Autodesk Inventor part; units mm, degrees
ref_plane "bolt_to_nut_XY" through (8, 0, 0) normal (1, 0, 0) x (0, 0, -1)
ref_plane "bolt_to_nut_YZ" through (8, 0, 0) normal (0, 0, -1) x (0, 1, 0)
ref_plane "bolt_to_nut_ZX" through (8, 0, 0) normal (0, 1, 0) x (1, 0, 0)
sketch "Sketch_1" plane through (0, 0, 0) normal (0, 0, 1) x (1, 0, 0)
  line L0 (8, 0) -> (-5, 0)
  line L1 (-5, 0) -> (-5, 3.75)
  line L2 (-5, 3.75) -> (-4.5, 4.25)
  line L3 (-4.5, 4.25) -> (0, 4.25)
  line L4 (0, 4.25) -> (0, 2.5)
  line L5 (0, 2.5) -> (7.5095, 2.5)
  line L6 (7.5095, 2.5) -> (8, 2.0095)
  line L7 (8, 2.0095) -> (8, 0)
  line L8 (8, 0) -> (-5, 0)
revolve "Revolution1" add sketch "Sketch_1" angle 360 about axis through (8, 0, 0) along (1, 0, 0)
thread "Thread1"
sketch "Sketch2" plane through (-5, 0, 0) normal (-1, 0, 0) x (0, 0, 1)
  point P0 (0, 0)
hole "Hole1" at (-5, 0, 0) direction (1, 0, 0) diameter 4 depth 2.5 tip angle 150
sketch "Sketch_3" plane through (-5, 0, 0) normal (1, 0, 0) x (0, 0, -1)
  line L0 (-2, -1.1547) -> (0, -2.3094)
  line L1 (0, -2.3094) -> (2, -1.1547)
  line L2 (2, -1.1547) -> (2, 1.1547)
  line L3 (2, 1.1547) -> (0, 2.3094)
  line L4 (0, 2.3094) -> (-2, 1.1547)
  line L5 (-2, 1.1547) -> (-2, -1.1547)
extrude "Extrusion1" cut sketch "Sketch_3" along normal blind 2.5
ref_plane "bolt_to_nut_XY" through (8, 0, 0) normal (1, 0, 0) x (0, 0, -1)
ref_plane "bolt_to_nut_YZ" through (8, 0, 0) normal (0, 0, -1) x (0, 1, 0)
ref_plane "bolt_to_nut_ZX" through (8, 0, 0) normal (0, 1, 0) x (1, 0, 0)
ref_plane "screw1_XY" through (0, 0, 0) normal (1, 0, 0) x (0, 0, -1)
ref_plane "screw1_YZ" through (0, 0, 0) normal (0, 0, -1) x (0, 1, 0)
ref_plane "screw1_ZX" through (0, 0, 0) normal (0, 1, 0) x (1, 0, 0)
properties part number "CB5-8" material "鋼、炭素鋼"
Check sheet for the modelled part. Datum: model origin and axes. Units: mm. A direction names the side the tool comes from. Give positions to 0.01 mm unless a question says otherwise; leave off trailing zeros. Write each loop counter-clockwise with the first axis right and the second up, starting at its lowest first coordinate (ties: lowest second). Pieces come first, ordered by that corner, then holes.
Item 1: Cross-section at A-A (x = -3.25). Enter the section's corners in (y, z).
Item 2: Cross-section at C-C (x = 4.25). Enter the section's corners in (y, z).
Item 3: Scan lines: L1, parallel to Y at x = -2.75, z = 1.25; L2, parallel to X at y = -1.5, z = 3; L3, parallel to Z at x = -2.5, y = 3.75. Record each from-to range of solid material in increasing order.
Item 4: Gauge pin test, flat ends, axial feed: pin 1 (1.5 mm diameter, centred on x = -1.5, y = -3, fed in from -Z); pin 2 (2 mm diameter, centred on x = 3, z = 2.5, fed in from +Y); pin 3 (3 mm diameter, centred on x = 2, y = -1.5, fed in from -Z). Record the tip position at first contact, or that the pin passes through.
Item 5: Access from +Z, -Z, +X, -X, +Y, -Y to the whole of each face (thin tool, end or side, straight path). Record for faces 5 (the face through (3.81, -0.54, -2.44)), 6 (the face through (-3.77, -1.74, -0.99)), 7 (the face through (-5, 2, -2)).
Item 6: Draft check along Z on faces 1 (the face through (-2.218, 2.285, 3.584)), 2 (the face through (8, 0, 0)), 3 (the face through (-4, 0, -2)), 4 (the face through (-3.77, 1.74, 0.99)). Enter one of: released by +Z, released by -Z, zero draft, split by the parting line, or undercut.
Item 7: Cross-section at B-B (x = -0.5). Enter the section's corners in (y, z), and give its area (3 significant figures).
Report:
1. outline: circle Ø8.5 at (0, 0); hole (-2.31, 0) - (-1.15, -2) - (1.15, -2) - (2.31, 0) - (1.15, 2) - (-1.15, 2) - close
2. outline: circle Ø5 at (0, 0)
3. L1: y = -4.06 to -1.59, 1.59 to 4.06
3. L2: x = -5 to 0
3. L3: z = -2 to 2
4. pin 1: stops at z = -3.61
4. pin 2: stops at y = 2
4. pin 3: stops at z = -2.5
5. face 5: +X
5. face 6: -X
5. face 7: +Z, -Z, -X, +Y, -Y
6. face 1: split by the parting line
6. face 2: zero draft
6. face 3: undercut
6. face 4: undercut
7. outline: circle Ø8.5 at (0, 0)
7. area: 56.7 mm2
